CAD build for the part. Positions are in the model's coordinates, mm. A direction names the side the tool comes from. Coordinates: 2 decimals unless noted, no trailing zeros. Write each loop counter-clockwise with the first axis right and the second up, starting at its lowest first coordinate (ties: lowest second). Pieces come first, ordered by that corner, then holes. Notation, with made-up numbers: (36.5, -38.75) - (92.5, -38.75) arc R21 cw to (92.5, -27.75) - close; hole circle Ø2 at (43.5, 53.25). An arc over 180 degrees is marked (long way). Answer in a Markdown table with one row per item. Add a question column.
Q1. Drill centre lines: line 1 along X through (y, z) = (3.25, -76); line 2 along Z through (x, y) = (-5.5, 1.15); line 3 along X through (y, z) = (3.75, -77). Where is each one in solid material? Low to high. Write a range as from..to.
Q2. Two-plate mould, pull along X, no slides. Class faces 3 (the cylindrical face through (-22.502, 3.754, -19.468)), 4 (the cylindrical face through (-34.19, 2.03, -70.28)), 5 (the flat face through (-24, 0, -38)): +X half, -X half, draft (parallel to the pull), parting line (faces both ways), or undercut.
Q3. Band-saw the part on A-A (x = -74). List the corners of the cut face in (y, z), and give its area (3 significant figures).
Q4. Pin check, flat tips, straight feed: pin 1 (2 mm diameter, centred on y = 1.5, z = -36.5, fed in from -X); pin 2 (1 mm diameter, centred on y = 2.5, z = -70, fed in from -X); pin 3 (1 mm diameter, centred on x = 7.5, y = 1, fed in from -Z). Stop position of each tip, or through.
Q5. Band-saw the part on B-B (x = 0). List the corners of the cut face in (y, z).
Q6. Band-saw the part on C-C (y = 0.95). State how many separate pieces and enclosed holes the cut face has, and give its area (3 significant figures).
Q7. 3-axis set-ups, long thin cutter, end or side, ignore diameter. For faces 1 (the conical face through (30.41, 3.33, -7.82)), 2 (the flat face through (-44, 2, -80)): which of +Z, -Z, +X, -X, +Y, -Y reach the whole face in a straight line?
Q8. Band-saw the part on D-D (x = -58). List the corners of the cut face in (y, z).
```python
from build123d import *

# Parameters (mm, degrees)
EXTRUDE_1_DEPTH     = 4
FILLET_1_R          = 30
FILLET_2_R          = 30
SKETCH_2_R          = 2.25
SKETCH_2_R_2        = 16
CUT_EXTRUDE_1_DEPTH = 4
SKETCH_3_R          = 4.2
CUT_EXTRUDE_2_DEPTH = 4
FILLET_3_R          = 5
SKETCH_4_R          = 1.65
CUT_EXTRUDE_3_DEPTH = 4
FILLET_4_R          = 10
FILLET_5_R          = 3
SKETCH_7_W          = 16
SKETCH_7_H          = 4
EXTRUDE_3_DEPTH     = 4
CUT_EXTRUDE_5_DEPTH = 4
FILLET_7_R          = 1
CHAMFER_1_SIZE      = 3.5
SKETCH_9_R          = 1.2
CUT_EXTRUDE_6_DEPTH = 10
SKETCH_10_R         = 1.5
CUT_EXTRUDE_7_DEPTH = 10


with BuildPart() as part:
    # 草图1 → 凸台-拉伸1 (new body)
    with BuildSketch(Plane(origin=(0, 0, 0), x_dir=(1, 0, 0), z_dir=(0, 1, 0))):
        with BuildLine():
            Line((-85, 80), (-35, 80))
            Line((-35, 80), (-35, 70))
            Line((-35, 70), (0, 36))
            ThreePointArc((0, 36), (25.455844123, -25.455844123), (-36, 0))
            Line((-36, 0), (-85, 70))
            Line((-85, 70), (-85, 80))
        make_face()
    extrude(amount=EXTRUDE_1_DEPTH)

    # 圆角1
    fillet_1_edges = [part.edges().sort_by_distance(p)[0] for p in [
        (0, 2, -36),
    ]]
    fillet(fillet_1_edges, radius=FILLET_1_R)

    # 圆角2
    fillet_2_edges = [part.edges().sort_by_distance(p)[0] for p in [
        (-36, 2, 0),
    ]]
    fillet(fillet_2_edges, radius=FILLET_2_R)

    # 草图2 → 切除-拉伸1 (cut)
    with BuildSketch(Plane(origin=(0, 4, 0), x_dir=(1, 0, 0), z_dir=(0, 1, 0))):
        with Locations(Location((-20.506096654, 20.506096654, 0), (0, 0, 270))):
            Circle(SKETCH_2_R)
        with Locations(Location((28.011848962, 7.505752308, 0), (0, 0, 270))):
            Circle(SKETCH_2_R)
        with Locations(Location((-7.505752308, -28.011848962, 0), (0, 0, 270))):
            Circle(SKETCH_2_R)
        with Locations(Location((0, 0, 0), (0, 0, 270))):
            Circle(SKETCH_2_R_2)
    extrude(amount=-CUT_EXTRUDE_1_DEPTH, mode=Mode.SUBTRACT)

    # 草图3 → 切除-拉伸2 (cut)
    with BuildSketch(Plane(origin=(0, 4, 0), x_dir=(1, 0, 0), z_dir=(0, 1, 0))):
        with Locations((-13.611805538, 13.611805538)):
            Circle(SKETCH_3_R)
    extrude(amount=-CUT_EXTRUDE_2_DEPTH, mode=Mode.SUBTRACT)

    # 圆角3
    fillet_3_edges = [part.edges().sort_by_distance(p)[0] for p in [
        (-9.473632004, 2, -12.893808462),
        (-12.893808462, 2, -9.473632004),
    ]]
    fillet(fillet_3_edges, radius=FILLET_3_R)

    # 草图4 → 切除-拉伸3 (cut)
    with BuildSketch(Plane(origin=(0, 4, 0), x_dir=(1, 0, 0), z_dir=(0, 1, 0))):
        with Locations(Location((-46, 76, 0), (0, 0, 270))):
            Circle(SKETCH_4_R)
        with Locations(Location((-74, 76, 0), (0, 0, 90))):
            Circle(SKETCH_4_R)
    extrude(amount=-CUT_EXTRUDE_3_DEPTH, mode=Mode.SUBTRACT)

    # 圆角4
    fillet_4_edges = [part.edges().sort_by_distance(p)[0] for p in [
        (-35, 2, -70),
        (-85, 2, -70),
    ]]
    fillet(fillet_4_edges, radius=FILLET_4_R)

    # 圆角5
    fillet_5_edges = [part.edges().sort_by_distance(p)[0] for p in [
        (-85, 2, -80),
        (-35, 2, -80),
    ]]
    fillet(fillet_5_edges, radius=FILLET_5_R)

    # 草图7 → 凸台-拉伸3 (add)
    with BuildSketch(Plane(origin=(0, 4, 0), x_dir=(1, 0, 0), z_dir=(0, 1, 0))):
        with Locations((-60, 82)):
            Rectangle(SKETCH_7_W, SKETCH_7_H)
    extrude(amount=-EXTRUDE_3_DEPTH)

    # 草图8 → 切除-拉伸5 (cut)
    with BuildSketch(Plane(origin=(0, 4, 0), x_dir=(1, 0, 0), z_dir=(0, 1, 0))):
        with BuildLine():
            Line((-50, 80), (-52, 80))
            ThreePointArc((-52, 80), (-51, 79), (-50, 80))
        make_face()
        with BuildLine():
            Line((-70, 80), (-68, 80))
            ThreePointArc((-68, 80), (-69, 79), (-70, 80))
        make_face()
    extrude(amount=-CUT_EXTRUDE_5_DEPTH, mode=Mode.SUBTRACT)

    # 圆角7
    fillet_7_edges = [part.edges().sort_by_distance(p)[0] for p in [
        (-52, 2, -84),
        (-68, 2, -84),
    ]]
    fillet(fillet_7_edges, radius=FILLET_7_R)

    # 倒角1
    # the kernel refuses this chamfer: 3.5 mm, written as the material it takes off along each edge
    with BuildSketch(Plane(origin=(-20.506096654, 0, -20.506096654), x_dir=(0, 0, 1), z_dir=(-1, 0, 0))) as chamfer_1_piece_1:
        Polygon((2.25 + CHAMFER_1_SIZE, 0), (2.25, CHAMFER_1_SIZE), (2.25, 0), align=None)
    revolve(axis=Axis((-20.506096654, 0, -20.506096654), (0, 1, 0)), mode=Mode.SUBTRACT)
    with BuildSketch(Plane(origin=(28.011848962, 0, -7.505752308), x_dir=(0, 0, 1), z_dir=(-1, 0, 0))) as chamfer_1_piece_2:
        Polygon((2.25 + CHAMFER_1_SIZE, 0), (2.25, CHAMFER_1_SIZE), (2.25, 0), align=None)
    revolve(axis=Axis((28.011848962, 0, -7.505752308), (0, 1, 0)), mode=Mode.SUBTRACT)
    with BuildSketch(Plane(origin=(-7.505752308, 0, 28.011848962), x_dir=(0, 0, 1), z_dir=(-1, 0, 0))) as chamfer_1_piece_3:
        Polygon((2.25 + CHAMFER_1_SIZE, 0), (2.25, CHAMFER_1_SIZE), (2.25, 0), align=None)
    revolve(axis=Axis((-7.505752308, 0, 28.011848962), (0, 1, 0)), mode=Mode.SUBTRACT)

    # 草图9 → 切除-拉伸6 (cut)
    with BuildSketch(Plane.XZ):
        with Locations(Location((-29.401166302, -40.007142113, 0), (0, 0, 270))):
            Circle(SKETCH_9_R)
        with Locations(Location((-43.686880588, -54.004226358, 0), (0, 0, 270))):
            Circle(SKETCH_9_R)
    extrude(amount=-CUT_EXTRUDE_6_DEPTH, mode=Mode.SUBTRACT)

    # 草图10 → 切除-拉伸7 (cut)
    with BuildSketch(Plane.XZ):
        with Locations(Location((-29.401166302, -40.007142113, 0), (0, 0, 270))):
            Circle(SKETCH_10_R)
        with Locations(Location((-43.686880588, -54.004226358, 0), (0, 0, 270))):
            Circle(SKETCH_10_R)
    extrude(amount=-CUT_EXTRUDE_7_DEPTH, mode=Mode.SUBTRACT)


solid = part.part
```
Checked values:
| question | item | result |
|---|---|---|
| 1 | line 1 | x = -85..-75.65, -72.35..-47.65, -44.35..-35 |
| 1 | line 2 | z = -41.47..-15.04, 15.02..23.87, 32.15..35.58 |
| 1 | line 3 | x = -85..-75.31, -72.69..-47.31, -44.69..-35 |
| 2 | face 3 | undercut |
| 2 | face 4 | +X half |
| 2 | face 5 | draft |
| 3 | outline | (0, -80) - (4, -80) - (4, -77.65) - (0, -77.65) - close; (0, -74.35) - (4, -74.35) - (4, -54.29) - (0, -54.29) - close |
| 3 | area | 89.7 mm² |
| 4 | pin 1 | stops at x = -62.25 |
| 4 | pin 2 | stops at x = -84.64 |
| 4 | pin 3 | stops at z = -35.32 |
| 5 | outline | (0, -37.86) - (4, -37.86) - (4, -16) - (0, -16) - close; (0, 16) - (4, 16) - (4, 36) - (0, 36) - close |
| 6 | separate pieces | 1 |
| 6 | enclosed holes | 8 |
| 6 | area | 6,150 mm² |
| 7 | face 1 | -Y |
| 7 | face 2 | -Z, +X, +Y, -Y |
| 8 | outline | (0, -84) - (4, -84) - (4, -31.43) - (0, -31.43) - close |
